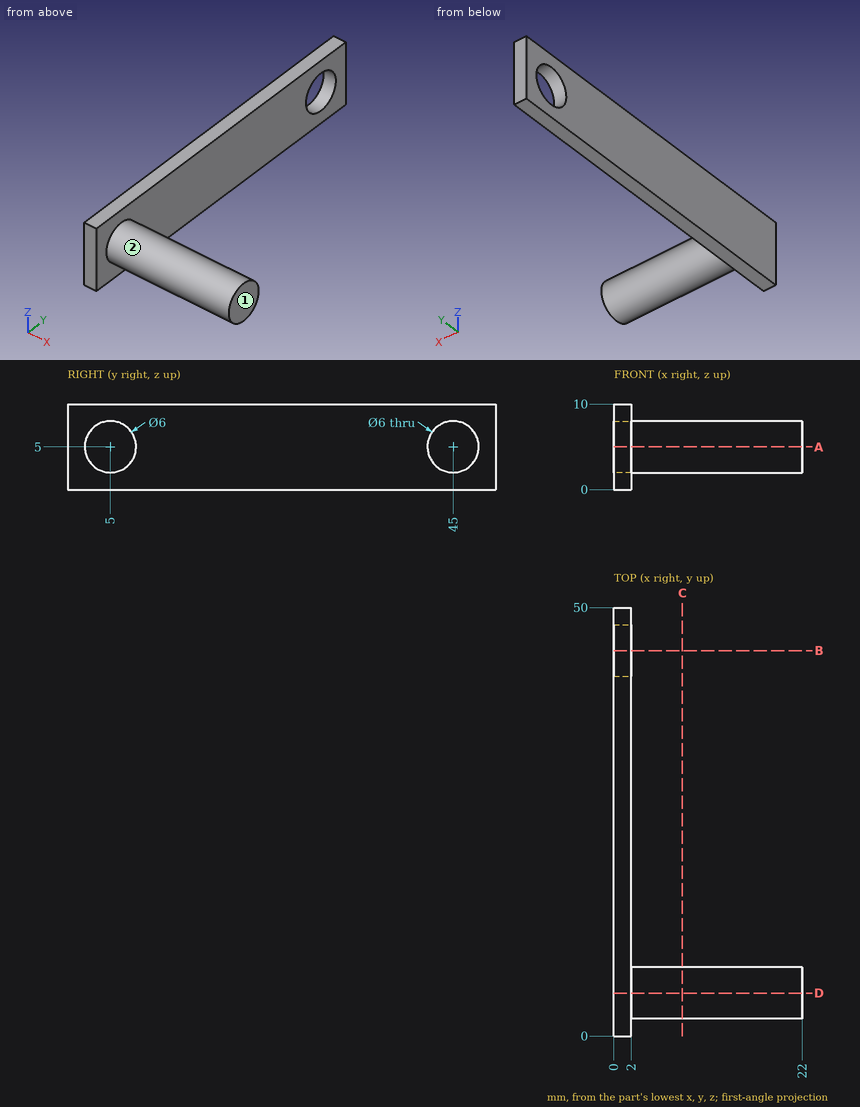
Job drawing, mm, ordinate dimensions from the low corner. One solid piece. A direction names the side the tool comes from. Round coordinates to 2 decimals unless told otherwise and drop trailing zeros. Loops run counter-clockwise (first coordinate to the right, second up) from the corner with the lowest first, then second, coordinate; pieces in that order, holes last. Notation, with made-up numbers: (5, 78.25) -> (21, 78.25) arc R28 ccw to (21, 103.25) -> close; hole circle Ø9 at (-38.75, 74.5). An arc over 180 degrees is marked (long way). Use a Markdown table: item, result.
1) Cut at B-B, the plane y = 45. List the corners of the cut face in (x, z), and give its area (3 significant figures).
The answers:
| item | result |
|---|---|
| outline | (0, 0) -> (2, 0) -> (2, 2) -> (0, 2) -> close; (0, 8) -> (2, 8) -> (2, 10) -> (0, 10) -> close |
| area | 8.00 mm2 |
2) Drop flat-ended pins along their axis: pin 1 Ø8 at (x, y) = (11.5, 9.5) entering from -Z; pin 2 Ø2 at (x, z) = (13.5, 3.5) entering from +Y; pin 3 Ø5 at (x, z) = (16, 9) entering from +Y. Give the stop position or say it passes through.
The answers:
| item | result |
|---|---|
| pin 1 | stops at z = 2.04 |
| pin 2 | stops at y = 7.96 |
| pin 3 | stops at y = 7.6 |
3) Cut at A-A, the plane z = 5. List the corners of the cut face in (x, y), and give its area (3 significant figures).
The answers:
| item | result |
|---|---|
| outline | (0, 0) -> (2, 0) -> (2, 2) -> (22, 2) -> (22, 8) -> (2, 8) -> (2, 42) -> (0, 42) -> close; (0, 48) -> (2, 48) -> (2, 50) -> (0, 50) -> close |
| area | 208 mm2 |
4) Cut at D-D, the plane y = 5. List the corners of the cut face in (x, z).
The answers:
| item | result |
|---|---|
| outline | (0, 0) -> (2, 0) -> (2, 2) -> (22, 2) -> (22, 8) -> (2, 8) -> (2, 10) -> (0, 10) -> close |
5) Cut at C-C, the plane x = 8. List the corners of the cut face in (y, z), and give its area (3 significant figures).
The answers:
| item | result |
|---|---|
| outline | circle Ø6 at (5, 5) |
| area | 28.3 mm2 |
6) Tool access for the marked faces 1 and 2: list every direction of +Z, -Z, +X, -X, +Y, -Y with a clear straight run to the whole face (end or side of a thin tool).
The answers:
| item | result |
|---|---|
| face 1 | +Z, -Z, +X, +Y, -Y |
| face 2 | +X |
7) Probe line 1 (Y direction, x = 0.45, z = 5); line 2 (X direction, y = 38.5, z = 6.75); line 3 (Z direction, x = 16.25, y = 3.5). List the from-to ranges inside material, lowest first. Write a range as [from, to].
The answers:
| item | result |
|---|---|
| line 1 | y = [0, 42], [48, 50] |
| line 2 | x = [0, 2] |
| line 3 | z = [2.4, 7.6] |
